Build history of the part. All positions in model axes, mm. Face numbers are marked on the shaded views. A direction names the side the tool comes from. Coordinates: 2 decimals unless noted, no trailing zeros. Order: outer loops, then holes, each group sorted by start corner. A loop starts at its lowest first (then second) coordinate and runs counter-clockwise, first axis right, second up. Notation, with made-up numbers: M 36.5,-37 L 60.5,-37 A28 ccw 60.5,-10 Z; hole C 11.5,-19.5 d8. An arc over 180 degrees is marked long. Write item = value, one per line. Start each with the question number.
Q1. 3-axis set-ups, long thin cutter, end or side, ignore diameter. For the marked faces 5 and 6: which of +Z, -Z, +X, -X, +Y, -Y reach the whole face in a straight line?
Q2. Band-saw the part on A-A on z = 35.15. Write the cut outline in (x, y), plus the area to 3 significant figures.
Q3. Band-saw the part on C-C on y = 7.75. Write the cut outline in (x, z), plus the area to 3 significant figures.
Q4. Band-saw the part on D-D on x = 31. Write the cut outline in (y, z).
Q5. Band-saw the part on B-B on x = 26.16. Write the cut outline in (y, z), plus the area to 3 significant figures.
Q6. Drill centre lines: probe 1 along X at (y, z) = (3.5, 9.5); probe 2 along X at (y, z) = (1.5, 35.15); probe 3 along Z at (x, y) = (29, 0.5). Where is each one in solid material? Low to high.
Q7. Pin check, flat tips, straight feed: P1, Ø20, axis at x = 26.16, z = 35.15, coming from the -Y side; P2, Ø5, axis at x = 9, z = 11.5, coming from the -Y side. Stop position of each tip, or through.
Q8. Pull direction X, two halves, no side cores. Call the marked faces 1, 2, 3 and 4: released by +X, released by -X, zero draft, split by the parting line, or undercut.
```python
from build123d import *

# Parameters (mm, degrees)
SKETCH2_W           = 40
SKETCH2_H           = 50
BOSS_EXTRUDE1_DEPTH = 10
SKETCH3_R           = 11.2
SKETCH3_R_2         = 7.5
CUT_EXTRUDE1_DEPTH  = 7
SKETCH4_R           = 7.5
SKETCH4_R_2         = 4.2
CUT_EXTRUDE2_DEPTH  = 65.807406984


with BuildPart() as part:
    # Sketch2 → Boss-Extrude1 (new body)
    with BuildSketch(Plane(origin=(0, 0, 0), x_dir=(1, 0, 0), z_dir=(0, 1, 0))):
        with Locations((20, -25)):
            Rectangle(SKETCH2_W, SKETCH2_H)
    extrude(amount=BOSS_EXTRUDE1_DEPTH)

    # Sketch3 → Cut-Extrude1 (cut)
    # profile 1 of 2: a face of its own
    with BuildSketch(Plane.XZ):
        with Locations(Location((26.16, 35.15, 0), (0, 0, 270))):
            Circle(SKETCH3_R)
        with Locations((26.16, 35.15)):
            Circle(SKETCH3_R_2, mode=Mode.SUBTRACT)
    # profile 2 of 2: a face of its own
    with BuildSketch(Plane.XZ):
        with Locations((26.16, 35.15)):
            Circle(SKETCH3_R_2)
    extrude(amount=-CUT_EXTRUDE1_DEPTH, mode=Mode.SUBTRACT)

    # Sketch4 → Cut-Extrude2 (cut, through all)
    with BuildSketch(Plane.XZ):
        with Locations(Location((26.16, 35.15, 0), (0, 0, 270))):
            Circle(SKETCH4_R)
        with Locations(Location((26.16, 9.5, 0), (0, 0, 270))):
            Circle(SKETCH4_R_2)
    extrude(amount=-CUT_EXTRUDE2_DEPTH, mode=Mode.SUBTRACT)


solid = part.part
```
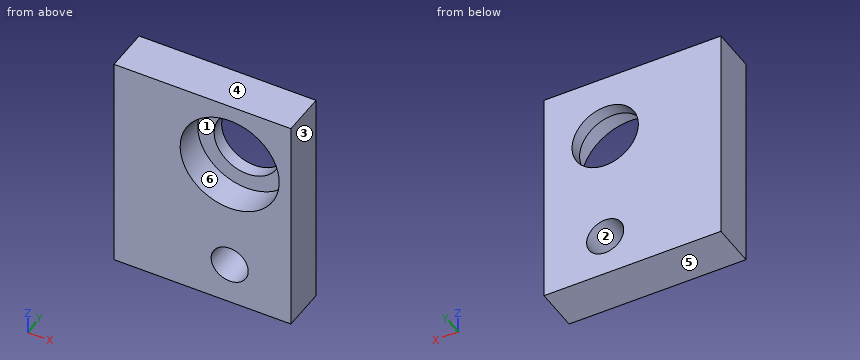
Recorded:
q1.face_5 = -Z, +X, -X, +Y, -Y
q1.face_6 = -Y
q2.outline = M 0,0 L 14.96,0 L 14.96,7 L 18.66,7 L 18.66,10 L 0,10 Z; M 33.66,7 L 37.36,7 L 37.36,0 L 40,0 L 40,10 L 33.66,10 Z
q2.area = 198 mm2
q3.outline = M 0,0 L 40,0 L 40,50 L 0,50 Z; hole C 26.16,35.15 d15; hole C 26.16,9.5 d8.4
q3.area = 1,770 mm2
q4.outline = M 0,0 L 10,0 L 10,29.42 L 7,29.42 L 7,25.05 L 0,25.05 Z; M 0,45.25 L 7,45.25 L 7,40.88 L 10,40.88 L 10,50 L 0,50 Z
q5.outline = M 0,0 L 10,0 L 10,5.3 L 0,5.3 Z; M 0,13.7 L 10,13.7 L 10,27.65 L 7,27.65 L 7,23.95 L 0,23.95 Z; M 0,46.35 L 7,46.35 L 7,42.65 L 10,42.65 L 10,50 L 0,50 Z
q5.area = 214 mm2
q6.probe_1 = 0 to 21.96, 30.36 to 40
q6.probe_2 = 0 to 14.96, 37.36 to 40
q6.probe_3 = 0 to 6.41, 12.59 to 24.32, 45.98 to 50
q7.P1 = 7
q7.P2 = 0
q8.face_1 = undercut
q8.face_2 = undercut
q8.face_3 = released by +X
q8.face_4 = zero draft
